```python
from build123d import *

# Parameters (mm, degrees)
F0_W     = 200
F0_H     = 100
F1_DEPTH = 25
F2_W     = 200
F2_H     = 15
F3_DEPTH = 20
F4_SIZE  = 0.5
F6_DEPTH = 1.5


with BuildPart() as f1:
    # F0 (on Top) → F1 (new body)
    with BuildSketch(Plane.XY):
        Rectangle(F0_W, F0_H)
    extrude(amount=-F1_DEPTH)

    # F2 (on face) → F3 (cut)
    with BuildSketch(Plane.XY):
        with Locations((0, 25.0000003725)):
            Rectangle(F2_W, F2_H)
        with Locations((0, -25.0000003725)):
            Rectangle(F2_W, F2_H)
    extrude(amount=-F3_DEPTH, mode=Mode.SUBTRACT)

    # F4
    f4_edges = [f1.edges().sort_by_distance(p)[0] for p in [
        (0, -50, 0),
        (0, -32.5, 0),
        (0, -17.5, 0),
        (0, 17.5, 0),
        (0, 32.5, 0),
        (0, 50, 0),
        (100, -41.25, 0),
        (100, 0, 0),
        (100, 41.25, 0),
        (-100, 41.25, 0),
        (-100, 0, 0),
        (-100, -41.25, 0),
    ]]
    chamfer(f4_edges, length=F4_SIZE)

    # F5 (on Top) → F6 (cut)
    with BuildSketch(Plane.XY):
        with BuildLine():
            Line((69, 55), (69, 45))
            Line((69, 45), (-69, 45))
            Line((-69, 45), (-69, 55))
            ThreePointArc((-69, 55), (-72, 58), (-75, 55))
            Line((-75, 55), (-75, -55))
            ThreePointArc((-75, -55), (-72, -52), (-69, -55))
            Line((-69, -55), (-69, -45))
            Line((-69, -45), (69, -45))
            Line((69, -45), (69, -55))
            ThreePointArc((69, -55), (72, -58), (75, -55))
            Line((75, -55), (75, 0))
            Line((75, 0), (75, 55))
            ThreePointArc((75, 55), (72, 58), (69, 55))
        make_face()
    extrude(amount=-F6_DEPTH, mode=Mode.SUBTRACT)


solid = f1.part
```
Check sheet for the modelled part. Datum: model origin and axes. Units: mm. A direction names the side the tool comes from. Give positions to 0.01 mm unless a question says otherwise; leave off trailing zeros. Write each loop counter-clockwise with the first axis right and the second up, starting at its lowest first coordinate (ties: lowest second). Pieces come first, ordered by that corner, then holes.
Item 1: Cross-section at D-D (x = 12.5). Enter the section's corners in (y, z).
Item 2: Cross-section at B-B (x = -78). Enter the section's corners in (y, z), and give its area (3 significant figures).
Item 3: Cross-section at A-A (z = -4.75). Enter the section's corners in (x, y), and give its area (3 significant figures).
Item 4: Draft check along X on faces 1 (the face through (100, -1, -13)), 2 (the face through (-100, -1, -13)), 3 (the face through (-1, 0, -1.5)), 4 (the face through (-1, 25, -20)). Enter one of: released by +X, released by -X, zero draft, split by the parting line, or undercut.
Item 5: Scan lines: L1, parallel to Y at x = -88, z = -10.75; L2, parallel to X at y = -41, z = -1.25; L3, parallel to Z at x = 6.5, y = -4. Record each from-to range of solid material in increasing order.
Item 6: Gauge pin test, flat ends, axial feed: pin 1 (8.5 mm diameter, centred on x = 23, y = 45.5, fed in from +Z); pin 2 (5 mm diameter, centred on x = 30.5, y = -6.5, fed in from +Z); pin 3 (1.5 mm diameter, centred on x = 12.5, y = 19, fed in from +Z). Record the tip position at first contact, or that the pin passes through.
Item 7: Cross-section at C-C (y = -36.5). Enter the section's corners in (x, z).
Item 8: Access from +Z, -Z, +X, -X, +Y, -Y to the whole of each face (thin tool, end or side, straight path). Record for faces 5 (the face through (87, -41, 0)), 6 (the face through (-1, 32.5, -10)).
Report:
1. outline: (-50, -25) - (50, -25) - (50, -0.5) - (49.5, 0) - (45, 0) - (45, -1.5) - (32.5, -1.5) - (32.5, -20) - (17.5, -20) - (17.5, -1.5) - (-17.5, -1.5) - (-17.5, -20) - (-32.5, -20) - (-32.5, -1.5) - (-45, -1.5) - (-45, 0) - (-49.5, 0) - (-50, -0.5) - close
2. outline: (-50, -25) - (50, -25) - (50, -0.5) - (49.5, 0) - (33, 0) - (32.5, -0.5) - (32.5, -20) - (17.5, -20) - (17.5, -0.5) - (17, 0) - (-17, 0) - (-17.5, -0.5) - (-17.5, -20) - (-32.5, -20) - (-32.5, -0.5) - (-33, 0) - (-49.5, 0) - (-50, -0.5) - close
2. area: 1,900 mm2
3. outline: (-100, -50) - (100, -50) - (100, -32.5) - (-100, -32.5) - close; (-100, -17.5) - (100, -17.5) - (100, 17.5) - (-100, 17.5) - close; (-100, 32.5) - (100, 32.5) - (100, 50) - (-100, 50) - close
3. area: 14,000 mm2
4. face 1: released by +X
4. face 2: released by -X
4. face 3: undercut
4. face 4: zero draft
5. L1: y = -50 to -32.5, -17.5 to 17.5, 32.5 to 50
5. L2: x = -100 to -75, 75 to 100
5. L3: z = -25 to -1.5
6. pin 1: stops at z = 0
6. pin 2: stops at z = -1.5
6. pin 3: stops at z = -20
7. outline: (-100, -25) - (100, -25) - (100, -0.5) - (99.5, 0) - (75, 0) - (75, -1.5) - (-75, -1.5) - (-75, 0) - (-99.5, 0) - (-100, -0.5) - close
8. face 5: +Z, +X, -X, +Y, -Y
8. face 6: +Z, +X, -X
